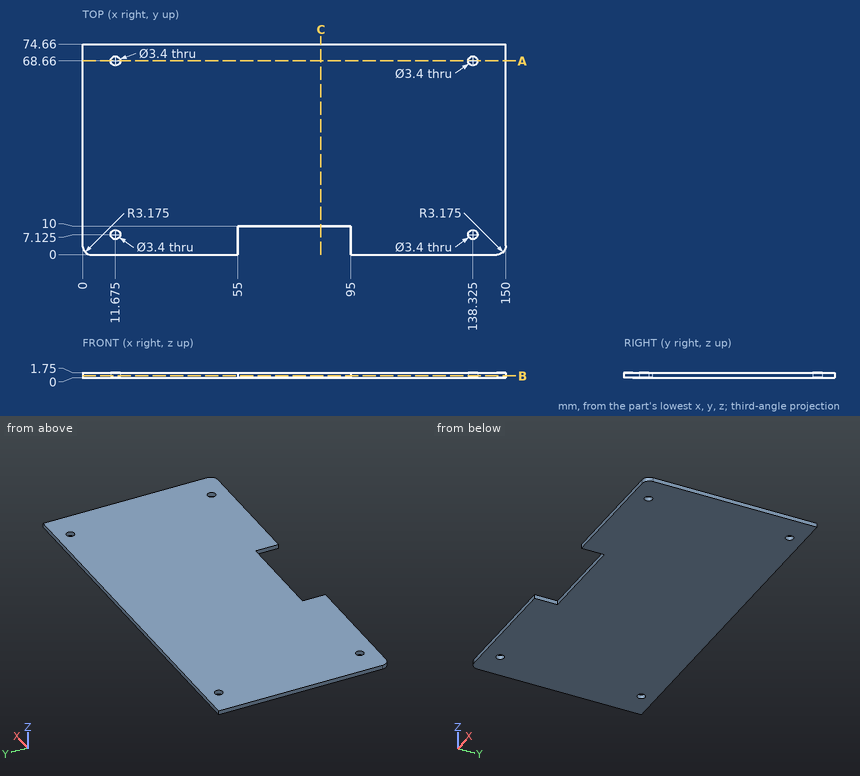
Drawing for the job (mm, zero at the part's lowest x, y, z). Round coordinates to 2 decimals unless told otherwise and drop trailing zeros. Loops run counter-clockwise (first coordinate to the right, second up) from the corner with the lowest first, then second, coordinate; pieces in that order, holes last. Notation, with made-up numbers: (1.25, 44.25) -> (5.25, 44.25) arc R21 cw to (5.25, 51.25) -> close; hole circle Ø3 at (38.25, 12.5). An arc over 180 degrees is marked (long way). Answer as CSV lines item,"result". Start each with the question number.
1) Probe line 1 along X through (y, z) = (68.66, 0.7) (3 decimals); line 2 along Y through (x, z) = (137, 0.9); line 3 along Y through (x, z) = (90, 1.45). List the from-to ranges inside material, lowest first.
2) Slice it at A-A (y = 68.66). List the corners of the cut face in (x, z) (3 decimals), plus the area to 3 significant figures.
3) Slice it at C-C (x = 84.5). List the corners of the cut face in (y, z), plus the area to 3 significant figures.
4) Slice it at B-B (z = 0.65). List the corners of the cut face in (x, y) (3 decimals).
5) Pin check, flat tip, straight feed: P1, Ø0.9, axis at x = 76.5, z = 1, coming from the -Y side. Stop position of the tip, or through.
Filled in:
1,line 1,"x = 0 to 9.975, 13.375 to 136.625, 140.025 to 150"
1,line 2,"y = 0 to 6.06, 8.19 to 67.59, 69.73 to 74.66"
1,line 3,"y = 10 to 74.66"
2,outline,"(0, 0) -> (9.975, 0) -> (9.975, 1.75) -> (0, 1.75) -> close; (13.375, 0) -> (136.625, 0) -> (136.625, 1.75) -> (13.375, 1.75) -> close; (140.025, 0) -> (150, 0) -> (150, 1.75) -> (140.025, 1.75) -> close"
2,area,"251 mm2"
3,outline,"(10, 0) -> (74.66, 0) -> (74.66, 1.75) -> (10, 1.75) -> close"
3,area,"113 mm2"
4,outline,"(0, 3.175) arc R3.175 ccw to (3.175, 0) -> (55, 0) -> (55, 10) -> (95, 10) -> (95, 0) -> (146.825, 0) arc R3.175 ccw to (150, 3.175) -> (150, 74.66) -> (0, 74.66) -> close; hole circle Ø3.4 at (11.675, 7.125); hole circle Ø3.4 at (11.675, 68.66); hole circle Ø3.4 at (138.325, 7.125); hole circle Ø3.4 at (138.325, 68.66)"
5,P1,"stops at y = 10"
